Geometry: final body of the model. Coordinates: model frame, mm. Face numbers are marked on the shaded views. Coordinates: 2 decimals unless noted, no trailing zeros. Loops run counter-clockwise (first coordinate to the right, second up) from the corner with the lowest first, then second, coordinate; pieces in that order, holes last. Notation, with made-up numbers: (19, 9.25) - (35, 9.25) arc R12 cw to (35, 14.25) - close; hole circle Ø4 at (28, 84.25). An arc over 180 degrees is marked (long way). Answer in a Markdown table with one row per item.
from build123d import *

# Parameters (mm, degrees)
BODY_START                   = 62.116699477
BODY_SHELL_OUTLINE_R         = 36.655940115
BODY_SHELL_DEPTH             = 30.774237315
BODY_SHELL_2_OUTLINE_R       = 37.655940115
BODY_SHELL_2_OUTLINE_R_2     = 36.655940115
BODY_SHELL_2_DEPTH           = 30.774237315
BASE_FILLET_R                = 5
PARTITION_EXTRUDE_DEPTH      = 2
PARTITION_EXTRUDE_DEPTH_BACK = 2
PARTITION_FILLET_1_R         = 2
PARTITION_FILLET_2_R         = 2


with BuildPart() as part:
    # Body Sketch → Body revolve (revolve)
    with BuildSketch(Plane.XY):
        Polygon((0, 0), (0, -112), (-25.3, -112), (-37.585940115, 62.116699477), (-36.655940115, 62.116699477), (-36.655940115, 92.890936792), (0, 92.890936792), align=None)
    revolve(axis=Axis((0, 0, 0), (0, -1, 0)))

    # Body Shell: read off the stored shape, not the designer's step
    # Body Shell outline → Body Shell (cut)
    with BuildSketch(Plane(origin=(0, 0, 0), x_dir=(1, 0, 0), z_dir=(0, 1, 0)).offset(BODY_START)):
        Circle(BODY_SHELL_OUTLINE_R)
    extrude(amount=BODY_SHELL_DEPTH, mode=Mode.SUBTRACT)

    # Body Shell 2 outline → Body Shell 2 (add)
    with BuildSketch(Plane(origin=(0, 0, 0), x_dir=(1, 0, 0), z_dir=(0, 1, 0)).offset(BODY_START)):
        Circle(BODY_SHELL_2_OUTLINE_R)
        Circle(BODY_SHELL_2_OUTLINE_R_2, mode=Mode.SUBTRACT)
    extrude(amount=BODY_SHELL_2_DEPTH)

    # Body Shell 3 outline → Body Shell 3 (revolve, cut)
    with BuildSketch(Plane.XY):
        Polygon((0, 62.116699477), (0, -117), (25.949678741, -117), (36.655940115, 34.729446569), (36.655940115, 62.116699477), align=None)
    revolve(axis=Axis((0, 0, 0), (0, 1, 0)), mode=Mode.SUBTRACT)

    # Body Shell 4 outline → Body Shell 4 (revolve)
    with BuildSketch(Plane.XY):
        Polygon((36.655940115, 62.116699477), (36.655940115, 34.729446569), (38.658988015, 63.116699477), (37.655940115, 63.116699477), (37.655940115, 62.116699477), align=None)
    revolve(axis=Axis((0, 0, 0), (0, 1, 0)))

    # Body Shell 5 outline → Body Shell 5 (revolve, cut)
    with BuildSketch(Plane.XY):
        Polygon((36.655940115, 62.116699477), (36.655940115, 48.936712516), (37.585940115, 62.116699477), align=None)
    revolve(axis=Axis((0, 0, 0), (0, 1, 0)), mode=Mode.SUBTRACT)

    # Body Shell 6 outline → Body Shell 6 (revolve)
    with BuildSketch(Plane.XY):
        Polygon((0, -112), (0, -117), (25.949678741, -117), (36.655940115, 34.729446569), (36.655940115, 48.936712516), (25.3, -112), align=None)
    revolve(axis=Axis((0, 0, 0), (0, 1, 0)))

    # Base Fillet
    base_fillet_edges = [part.edges().sort_by_distance(p)[0] for p in [
        (-25.949678741, -117, 0),
    ]]
    fillet(base_fillet_edges, radius=BASE_FILLET_R)

    # Partition Sketch → Partition Extrude (add, two sides: drawn at the far end of the back side and taken through both)
    with BuildSketch(Plane(origin=(0, 0, 0), x_dir=(0, 0, -1), z_dir=(1, 0, 0)).offset(-PARTITION_EXTRUDE_DEPTH_BACK)):
        Polygon((-25.32, -112.351932597), (25.32, -112.351932597), (26.77, -91.851932597), (-26.77, -91.851932597), align=None)
    extrude(amount=PARTITION_EXTRUDE_DEPTH + PARTITION_EXTRUDE_DEPTH_BACK)

    # Partition Fillet 1
    partition_fillet_1_edges = [part.edges().sort_by_distance(p)[0] for p in [
        (2, -91.851932597, 0),
    ]]
    fillet(partition_fillet_1_edges, radius=PARTITION_FILLET_1_R)

    # Partition Fillet 2
    partition_fillet_2_edges = [part.edges().sort_by_distance(p)[0] for p in [
        (-2, -91.851932597, 0),
    ]]
    fillet(partition_fillet_2_edges, radius=PARTITION_FILLET_2_R - 0.0001)  # a hair under: the kernel refuses the full size


solid = part.part
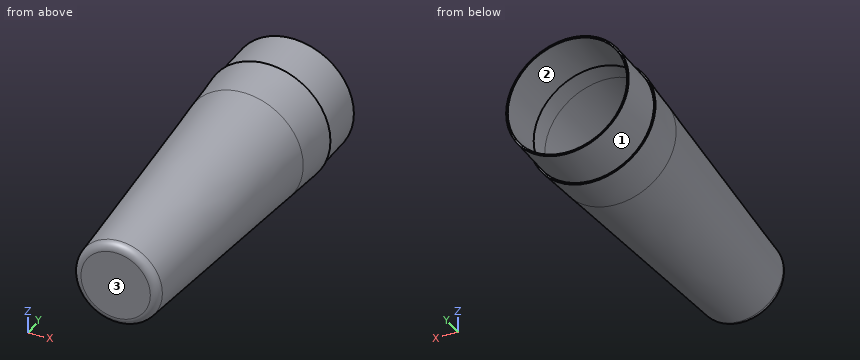
(1) Pull-direction query (X, two-part tool) for the marked faces 1, 2 and 3; classes: pulls with the +X half, pulls with the -X half, needs draft (parallel to the pull), parting line crosses it, or undercut.
Verdict:
| item | result |
|---|---|
| face 1 | parting line crosses it |
| face 2 | undercut |
| face 3 | needs draft |
(2) Cut plane A-A on y = -34. Output: boundary loops of the cut face in (x, z).
Verdict:
| item | result |
|---|---|
| outline | circle Ø63.61 at (0, 0); hole circle Ø61.61 at (0, 0) |
(3) Ray query, probe 1 along Z at (x, y) = (0, 79); probe 2 along Z at (x, y) = (-1, 70.5). Return the intervals inside material, ascending.
Verdict:
| item | result |
|---|---|
| probe 1 | z = -37.66 to -36.66, 36.66 to 37.66 |
| probe 2 | z = -37.64 to -36.64, 36.64 to 37.64 |
(4) First-contact query: pin 1 Ø5.5 at (y, z) = (-105, 2.5) entering from +X; pin 2 Ø10 at (y, z) = (-56, -5.5) entering from +X; pin 3 Ø5 at (x, y) = (-14.5, -77) entering from -Z. Flat tips, straight axial feed; report the tip coordinate or a pass-through.
Verdict:
| item | result |
|---|---|
| pin 1 | stops at x = 26.94 |
| pin 2 | stops at x = 30.44 |
| pin 3 | stops at z = -26.17 |
(5) Cut plane B-B on y = 23. Output: boundary loops of the cut face in (x, z), then the cut area to 3 significant figures.
Verdict:
| item | result |
|---|---|
| outline | circle Ø71.66 at (0, 0); hole circle Ø69.65 at (0, 0) |
| area | 223 mm² |
